For this review, take the finished solid that the model builds, in its own axes (mm). A direction names the side the tool comes from. Give positions to 0.01 mm unless a question says otherwise; leave off trailing zeros. Write each loop counter-clockwise with the first axis right and the second up, starting at its lowest first coordinate (ties: lowest second). Pieces come first, ordered by that corner, then holes. Notation, with made-up numbers: (61.5, -5.75) -> (80.5, -5.75) arc R12 cw to (80.5, 5.25) -> close; hole circle Ø5 at (-18, 59.25). An arc over 180 degrees is marked (long way). Answer as CSV lines item,"result".
```python
from build123d import *

# Parameters (mm, degrees)
SKETCH_1_R          = 20
SKETCH_1_R_2        = 7
EXTRUDE_1_DEPTH     = 10
EXTRUDE_START       = -10
EXTRUDE_2_DEPTH     = 10
SKETCH_3_R          = 7
EXTRUDE_3_DEPTH     = 10
CUT_EXTRUDE_START   = -5
SKETCH_4_R          = 7
CUT_EXTRUDE_1_DEPTH = 5


with BuildPart() as part:
    # 草图1 → 凸台-拉伸1 (new body)
    # profile 1 of 3: a face of its own
    with BuildSketch(Plane(origin=(0, 0, 0), x_dir=(1, 0, 0), z_dir=(0, 1, 0))):
        Circle(SKETCH_1_R)
        with Locations(Location((0, 0, 0), (0, 0, 270))):
            Circle(SKETCH_1_R_2, mode=Mode.SUBTRACT)
    # profile 2 of 3: a face of its own
    with BuildSketch(Plane(origin=(0, 0, 0), x_dir=(1, 0, 0), z_dir=(0, 1, 0))):
        with BuildLine():
            Line((0, -20), (88, -20))
            ThreePointArc((88, -20), (68, 0), (88, 20))
            Line((88, 20), (-1.4e-08, 20))
            ThreePointArc((-1.4e-08, 20), (14.142135619, 14.142135629), (20, 0))
            ThreePointArc((20, 0), (14.142135624, -14.142135624), (0, -20))
        make_face()
    # profile 3 of 3: a face of its own
    with BuildSketch(Plane(origin=(0, 0, 0), x_dir=(1, 0, 0), z_dir=(0, 1, 0))):
        with Locations((88, 0)):
            Circle(SKETCH_1_R)
        with Locations(Location((88, 0, 0), (0, 0, 270))):
            Circle(SKETCH_1_R_2, mode=Mode.SUBTRACT)
    extrude(amount=EXTRUDE_1_DEPTH)

    # 草图2 → 凸台-拉伸2 (add)
    with BuildSketch(Plane(origin=(0, 10, 0), x_dir=(1, 0, 0), z_dir=(0, 1, 0)).offset(EXTRUDE_START)):
        with BuildLine():
            Line((88, -20), (101.910822615, -20))
            Line((101.910822615, -20), (119.744098688, -11.302130098))
            ThreePointArc((119.744098688, -11.302130098), (175.999613382, 24.015412746), (242.422587784, 24))
            Line((242.422587784, 24), (245.659989933, 39.669053173))
            Line((245.659989933, 39.669053173), (232, 48))
            add(Edge.make_bspline(
                [(44, 20), (135.765778064, 51.236254285), (232, 48)],
                knots=[0, 0, 0, 1, 1, 1], degree=2))
            Line((44, 20), (88, 20))
            ThreePointArc((88, 20), (108, 0), (88, -20))
        make_face()
    extrude(amount=EXTRUDE_2_DEPTH)

    # 草图3 → 凸台-拉伸3 (add)
    with BuildSketch(Plane(origin=(0, 10, 0), x_dir=(1, 0, 0), z_dir=(0, 1, 0))):
        with BuildLine():
            Line((245.659989933, 39.669053173), (232, 48))
            add(Edge.make_bspline(
                [(232, 48), (135.765778064, 51.236254285), (44, 20)],
                knots=[0, 0, 0, 1, 1, 1], degree=2))
            Line((44, 20), (0, 20))
            ThreePointArc((0, 20), (-20, 0), (0, -20))
            Line((0, -20), (101.910822615, -20))
            Line((101.910822615, -20), (119.744098688, -11.302130098))
            ThreePointArc((119.744098688, -11.302130098), (175.999613382, 24.015412746), (242.422587784, 24))
            Line((242.422587784, 24), (245.659989933, 39.669053173))
        make_face()
        with Locations(Location((88, 0, 0), (0, 0, 270))):
            Circle(SKETCH_3_R, mode=Mode.SUBTRACT)
        with Locations(Location((0, 0, 0), (0, 0, 270))):
            Circle(SKETCH_3_R, mode=Mode.SUBTRACT)
    extrude(amount=EXTRUDE_3_DEPTH)

    # 草图4 → 切除-拉伸1 (cut)
    with BuildSketch(Plane(origin=(0, 20, 0), x_dir=(1, 0, 0), z_dir=(0, 1, 0)).offset(CUT_EXTRUDE_START)):
        with BuildLine():
            Line((242.422587784, 24), (245.659989933, 39.669053173))
            Line((245.659989933, 39.669053173), (232, 48))
            add(Edge.make_bspline(
                [(232, 48), (135.765778061, 51.236254285), (43.999999994, 19.999999998)],
                knots=[0, 0, 0, 1, 1, 1], degree=2))
            Line((43.999999994, 19.999999998), (0, 20))
            ThreePointArc((0, 20), (-20, 0), (0, -20))
            Line((0, -20), (101.910822615, -20))
            Line((101.910822615, -20), (119.744098688, -11.302130098))
            ThreePointArc((119.744098688, -11.302130098), (175.999613382, 24.015412746), (242.422587784, 24))
        make_face()
        with Locations(Location((0, 0, 0), (0, 0, 270))):
            Circle(SKETCH_4_R, mode=Mode.SUBTRACT)
        with Locations(Location((88, 0, 0), (0, 0, 270))):
            Circle(SKETCH_4_R, mode=Mode.SUBTRACT)
    extrude(amount=CUT_EXTRUDE_1_DEPTH, mode=Mode.SUBTRACT)


solid = part.part
```
Q1. Add section C-C (z = 14). Write out the cut boundary in (x, y), plus the area to 3 significant figures.
Answer block:
outline,"(-14.28, 0) -> (114.21, 0) -> (114.21, 15) -> (-14.28, 15) -> close"
area,"1,930 mm2"
Q2. Clearance check with flat-ended pins moving along their axes: pin 1 (12.5 mm diameter, centred on x = 88, z = 0, fed in from -Y); pin 2 (2 mm diameter, centred on y = 8.5, z = -2, fed in from +X). State where each tip first meets the part, or that it passes through.
Answer block:
pin 1,"passes through"
pin 2,"stops at x = 134.98"
Q3. To check wall thickness, follow probe 1 along X at (y, z) = (9, 0); probe 2 along X at (y, z) = (1.25, 1); probe 3 along Z at (x, y) = (83, 9.75). State the ranges of each line that lie inside material, in increasing order. Write a range as [from, to].
Answer block:
probe 1,"x = [-20, -7], [7, 81], [95, 131.32]"
probe 2,"x = [-19.97, -6.93], [6.93, 81.07], [94.93, 130.16]"
probe 3,"z = [-31.67, -4.9], [4.9, 20]"
Q4. Add section B-B (y = 5.5). State how many separate pieces and enclosed holes the cut face has, plus the area to 3 significant figures.
Answer block:
separate pieces,"1"
enclosed holes,"2"
area,"9,140 mm2"
Q5. For faces 4 (the cylindrical face through (-6.834, 7.395, -1.517)), 5 (the flat face through (22, 7, -20)), list the 3-axis set-ups (+Z, -Z, +X, -X, +Y, -Y) from which the entire face can be reached by the end or side of a thin tool; tool diameter is ignored.
Answer block:
face 4,"+Y, -Y"
face 5,"-Z, -X, +Y, -Y"
Q6. Add section A-A (z = 0). Write out the cut boundary in (x, y).
Answer block:
outline,"(-20, 0) -> (-7, 0) -> (-7, 15) -> (-20, 15) -> close; (7, 0) -> (81, 0) -> (81, 15) -> (7, 15) -> close; (95, 0) -> (131.32, 0) -> (131.32, 15) -> (95, 15) -> close"
Q7. Draft analysis for pull direction Z (two halves, no side actions). For faces 1 (the flat face through (110.703, 7.395, 15.712)), 2 (the flat face through (238.926, 7.395, -43.776)), 3 (the cylindrical face through (94.94, 7.4, -0.91)), state which applies: released by +Z, released by -Z, zero draft, split by the parting line, or undercut.
Answer block:
face 1,"released by +Z"
face 2,"released by -Z"
face 3,"undercut"
